from build123d import *

# Parameters (mm, degrees)
F0_W      = 87
F0_H      = 87
F1_DEPTH  = 5
F3_DEPTH  = 5
F6_D      = 6.5
F8_DEPTH  = 15
F9_R      = 12.5
F10_DEPTH = 5


with BuildPart() as f1:
    # F0 (on Top) → F1 (new body)
    with BuildSketch(Plane.XY):
        Rectangle(F0_W, F0_H)
    extrude(amount=F1_DEPTH)

    # F2 (on face) → F3 (join)
    with BuildSketch(Plane.XY.offset(5)):
        with BuildLine():
            ThreePointArc((-17.67767, 17.67767), (-15.821292, 19.356826), (-13.806304, 20.841928))
            ThreePointArc((-13.806304, 20.841928), (-21.213203, 21.213203), (-20.841928, 13.806304))
            ThreePointArc((-20.841928, 13.806304), (-19.356826, 15.821292), (-17.67767, 17.67767))
        make_face()
        with BuildLine():
            ThreePointArc((-20.841928, 13.806304), (-17.427356, 12.683939), (-14.142136, 14.142136))
            Line((-14.142136, 14.142136), (-17.67767, 17.67767))
            ThreePointArc((-17.67767, 17.67767), (-19.356826, 15.821292), (-20.841928, 13.806304))
        make_face()
        with BuildLine():
            ThreePointArc((-12.67767, 17.67767), (-12.968273, 19.357428), (-13.806304, 20.841928))
            ThreePointArc((-13.806304, 20.841928), (-15.821292, 19.356826), (-17.67767, 17.67767))
            Line((-17.67767, 17.67767), (-14.142136, 14.142136))
            ThreePointArc((-14.142136, 14.142136), (-13.058272, 15.764252), (-12.67767, 17.67767))
        make_face()
        with BuildLine():
            ThreePointArc((-12.67767, -17.67767), (-13.058272, -15.764252), (-14.142136, -14.142136))
            Line((-14.142136, -14.142136), (-17.67767, -17.67767))
            ThreePointArc((-17.67767, -17.67767), (-15.821292, -19.356826), (-13.806304, -20.841928))
            ThreePointArc((-13.806304, -20.841928), (-12.968273, -19.357428), (-12.67767, -17.67767))
        make_face()
        with BuildLine():
            Line((-17.67767, -17.67767), (-14.142136, -14.142136))
            ThreePointArc((-14.142136, -14.142136), (-17.427356, -12.683939), (-20.841928, -13.806304))
            ThreePointArc((-20.841928, -13.806304), (-19.356826, -15.821292), (-17.67767, -17.67767))
        make_face()
        with BuildLine():
            ThreePointArc((-20.841928, -13.806304), (-21.213203, -21.213203), (-13.806304, -20.841928))
            ThreePointArc((-13.806304, -20.841928), (-15.821292, -19.356826), (-17.67767, -17.67767))
            ThreePointArc((-17.67767, -17.67767), (-19.356826, -15.821292), (-20.841928, -13.806304))
        make_face()
        with BuildLine():
            ThreePointArc((13.806304, -20.841928), (15.821292, -19.356826), (17.67767, -17.67767))
            Line((17.67767, -17.67767), (14.142136, -14.142136))
            ThreePointArc((14.142136, -14.142136), (12.683939, -17.427356), (13.806304, -20.841928))
        make_face()
        with BuildLine():
            ThreePointArc((17.67767, -17.67767), (19.356826, -15.821292), (20.841928, -13.806304))
            ThreePointArc((20.841928, -13.806304), (17.427356, -12.683939), (14.142136, -14.142136))
            Line((14.142136, -14.142136), (17.67767, -17.67767))
        make_face()
        with BuildLine():
            ThreePointArc((22.67767, -17.67767), (22.195484, -15.535392), (20.841928, -13.806304))
            ThreePointArc((20.841928, -13.806304), (19.356826, -15.821292), (17.67767, -17.67767))
            ThreePointArc((17.67767, -17.67767), (15.821292, -19.356826), (13.806304, -20.841928))
            ThreePointArc((13.806304, -20.841928), (19.357428, -22.387066), (22.67767, -17.67767))
        make_face()
        with BuildLine():
            ThreePointArc((17.67767, 17.67767), (19.356826, 15.821292), (20.841928, 13.806304))
            ThreePointArc((20.841928, 13.806304), (22.195484, 15.535392), (22.67767, 17.67767))
            ThreePointArc((22.67767, 17.67767), (19.357428, 22.387066), (13.806304, 20.841928))
            ThreePointArc((13.806304, 20.841928), (15.821292, 19.356826), (17.67767, 17.67767))
        make_face()
        with BuildLine():
            ThreePointArc((14.142136, 14.142136), (17.427356, 12.683939), (20.841928, 13.806304))
            ThreePointArc((20.841928, 13.806304), (19.356826, 15.821292), (17.67767, 17.67767))
            Line((17.67767, 17.67767), (14.142136, 14.142136))
        make_face()
        with BuildLine():
            Line((14.142136, 14.142136), (17.67767, 17.67767))
            ThreePointArc((17.67767, 17.67767), (15.821292, 19.356826), (13.806304, 20.841928))
            ThreePointArc((13.806304, 20.841928), (12.683939, 17.427356), (14.142136, 14.142136))
        make_face()
    extrude(amount=F3_DEPTH)

    # F6 (through all)
    with Locations(Plane.XY.offset(10)):
        with Locations((-17.67767, 17.67767), (17.67767, 17.67767), (17.67767, -17.67767), (-17.67767, -17.67767)):
            Hole(F6_D / 2)

    # F7 (on face) → F8 (join)
    with BuildSketch(Plane.XY.offset(5)):
        with BuildLine():
            ThreePointArc((-43.5, 38), (-38, 32.5), (-32.5, 38))
            ThreePointArc((-32.5, 38), (-34.110913, 41.889087), (-38, 43.5))
            ThreePointArc((-38, 43.5), (-41.889087, 41.889087), (-43.5, 38))
        make_face()
        with BuildLine():
            ThreePointArc((-32.5, -38), (-38, -32.5), (-43.5, -38))
            ThreePointArc((-43.5, -38), (-41.889087, -41.889087), (-38, -43.5))
            ThreePointArc((-38, -43.5), (-34.110913, -41.889087), (-32.5, -38))
        make_face()
        with BuildLine():
            ThreePointArc((38, -43.5), (41.889087, -41.889087), (43.5, -38))
            ThreePointArc((43.5, -38), (34.110913, -34.110913), (38, -43.5))
        make_face()
    extrude(amount=F8_DEPTH)

    # F9 (on face) → F10 (cut)
    with BuildSketch(Plane.XY.offset(5)):
        Polygon((5.01014, 39.079089), (5.01014, 26.55374), (15.030419, 26.55374), (25.050698, 39.079089), align=None)
        Polygon((-5.01014, 39.079089), (-25.050698, 39.079089), (-15.030419, 26.55374), (-5.01014, 26.55374), align=None)
        Polygon((26.55374, 15.030419), (26.55374, 5.01014), (39.079089, 5.01014), (39.079089, 25.050698), align=None)
        Polygon((39.079089, -5.01014), (26.55374, -5.01014), (26.55374, -15.030419), (39.079089, -25.050698), align=None)
        Polygon((-15.030419, -26.55374), (-25.050698, -39.079089), (-5.01014, -39.079089), (-5.01014, -26.55374), align=None)
        Polygon((5.01014, -26.55374), (5.01014, -39.079089), (25.050698, -39.079089), (15.030419, -26.55374), align=None)
        Polygon((-26.55374, 5.01014), (-26.55374, 15.030419), (-39.079089, 25.050698), (-39.079089, 5.01014), align=None)
        Polygon((-26.55374, -5.01014), (-39.079089, -5.01014), (-39.079089, -25.050698), (-26.55374, -15.030419), align=None)
        Circle(F9_R)
    extrude(amount=-F10_DEPTH, mode=Mode.SUBTRACT)


solid = f1.part
Could you check a few things on this model? Use its own coordinates, in mm. A direction names the side the tool comes from. Give positions to 0.01 mm unless a question says otherwise; leave off trailing zeros. Write each loop counter-clockwise with the first axis right and the second up, starting at its lowest first coordinate (ties: lowest second). Pieces come first, ordered by that corner, then holes. Notation, with made-up numbers: (35.5, 69) -> (86.5, 69) arc R14 ccw to (86.5, 81) -> close; hole circle Ø4 at (-26.75, 84). An arc over 180 degrees is marked (long way). Write each question's results on one line, items separated by ' | '. Start each with the question number.
Q1. We'd pull the mould along X, two halves only. Please class faces 3 (the face through (-14, -18, 10)), 4 (the face through (11.923, 3.755, 2.535)): +X half, -X half, draft (parallel to the pull), parting line (faces both ways), or undercut.
Q2. I'm going to push flat-ended pins straight in: pin 1 Ø5 at (x, y) = (15.5, 16.5) entering from +Z; pin 2 Ø1.5 at (x, y) = (21, -29) entering from +Z. Where does each tip first touch, or does it pass through?
Q3. Suppose I cut it at D-D, the plane y = -16.5. List the corners of the cut face in (x, z) for me.
Q4. Suppose I cut it at C-C, the plane z = 14.5. List the corners of the cut face in (x, y) for me, and give its area (3 significant figures).
Q5. I need wall thicknesses on probe 1 along Y at (x, z) = (17.5, 9); probe 2 along Y at (x, z) = (-9.5, 2.75); probe 3 along Z at (x, y) = (14, 21.5). Which ranges of each line are inside material? Lowest first, please.
Q6. Suppose I cut it at A-A, the plane y = 0. List the corners of the cut face in (x, z) for me, and give its area (3 significant figures).
Q7. Suppose I cut it at B-B, the plane x = -10. List the corners of the cut face in (y, z) for me, and give its area (3 significant figures).
Q8. Which directions (+Z, -Z, +X, -X, +Y, -Y) give clear straight access to the entire face, cutting with the end or side of a thin tool? Please do faces 1 (the face through (-10, 26.554, 3)), 2 (the face through (19, -21, 10)).
Outcome:
1) face 3: draft | face 4: undercut
2) pin 1: z = 10 | pin 2: z = 5
3) outline: (-43.5, 0) -> (-39.08, 0) -> (-39.08, 5) -> (-43.5, 5) -> close; (-28.39, 0) -> (-20.71, 0) -> (-20.71, 10) -> (-22.54, 10) -> (-22.54, 5) -> (-28.39, 5) -> close; (-14.65, 0) -> (14.65, 0) -> (14.65, 10) -> (12.82, 10) -> (12.82, 5) -> (-12.82, 5) -> (-12.82, 10) -> (-14.65, 10) -> close; (20.71, 0) -> (28.39, 0) -> (28.39, 5) -> (22.54, 5) -> (22.54, 10) -> (20.71, 10) -> close; (39.08, 0) -> (43.5, 0) -> (43.5, 5) -> (39.08, 5) -> close
4) outline: (-43.5, -38) arc R5.5 ccw to (-38, -43.5) arc R5.5 ccw to (-32.5, -38) arc R5.5 ccw to start; (-43.5, 38) arc R5.5 ccw to (-32.5, 38) arc R5.5 ccw to (-38, 43.5) arc R5.5 ccw to start; (38, -43.5) arc R5.5 ccw to (43.5, -38) arc R5.5 ccw (long way) to start | area: 285 mm2
5) probe 1: -22.67 to -20.92, -14.43 to -12.68, 12.68 to 14.43, 20.92 to 22.67 | probe 2: -43.5 to -39.08, -26.55 to -8.12, 8.12 to 26.55, 39.08 to 43.5 | probe 3: 0 to 5
6) outline: (-43.5, 0) -> (-12.5, 0) -> (-12.5, 5) -> (-43.5, 5) -> close; (12.5, 0) -> (43.5, 0) -> (43.5, 5) -> (12.5, 5) -> close | area: 310 mm2
7) outline: (-43.5, 0) -> (-39.08, 0) -> (-39.08, 5) -> (-43.5, 5) -> close; (-26.55, 0) -> (-7.5, 0) -> (-7.5, 5) -> (-26.55, 5) -> close; (7.5, 0) -> (26.55, 0) -> (26.55, 5) -> (7.5, 5) -> close; (39.08, 0) -> (43.5, 0) -> (43.5, 5) -> (39.08, 5) -> close | area: 235 mm2
8) face 1: +Z, -Z | face 2: +Z, +X, -X, +Y, -Y
